Build history of the part. All positions in model axes, mm. A direction names the side the tool comes from. Round coordinates to 2 decimals unless told otherwise and drop trailing zeros. Loops run counter-clockwise (first coordinate to the right, second up) from the corner with the lowest first, then second, coordinate; pieces in that order, holes last. Notation, with made-up numbers: M -34,41 L -10,41 A24 ccw -10,67 Z; hole C 73,36 d11. An arc over 180 degrees is marked long. One line per item, written item: value.
```python
from build123d import *

# Parameters (mm, degrees)
SKETCH_2_W               = 50
SKETCH_2_H               = 4
EXTRUDE_2_DEPTH          = 22.5
SKETCH_15_R              = 1.4
EXTRUDE_8_DEPTH          = 5
SKETCH_3_W               = 30
SKETCH_3_H               = 20
EXTRUDE_4_DEPTH          = 20
EXTRUDE_9_DEPTH          = 17.5
EXTRUDE_10_DEPTH         = 15
CUT_EXTRUDE_1_REACH      = 58.089
SKETCH_19_R              = 2.1
SKETCH_20_R              = 2
CUT_EXTRUDE_2_DEPTH      = 10
CUT_EXTRUDE_3_DEPTH      = 70.524879929
CUT_EXTRUDE_3_DEPTH_BACK = 70.524879929


with BuildPart() as part:
    # 草圖2 → 填料-伸長2 (new, symmetric)
    with BuildSketch(Plane(origin=(0, 0, 0), x_dir=(0, 0, -1), z_dir=(1, 0, 0))):
        with Locations((25, 2)):
            Rectangle(SKETCH_2_W, SKETCH_2_H)
    extrude(amount=EXTRUDE_2_DEPTH, both=True)

    # 草圖15 → 填料-伸長8 (add)
    with BuildSketch(Plane(origin=(0, 4, 0), x_dir=(1, 0, 0), z_dir=(0, 1, 0))):
        with Locations(Location((17.5, 39.2, 0), (0, 0, 90))):
            Circle(SKETCH_15_R)
        with Locations(Location((17.5, 24.2, 0), (0, 0, 90))):
            Circle(SKETCH_15_R)
    extrude(amount=EXTRUDE_8_DEPTH)

    # 草圖3 → 填料-伸長4 (add)
    with BuildSketch(Plane(origin=(0, 4, 0), x_dir=(1, 0, 0), z_dir=(0, 1, 0))):
        with Locations((0, 10)):
            Rectangle(SKETCH_3_W, SKETCH_3_H)
    extrude(amount=EXTRUDE_4_DEPTH)

    # 草圖16 → 填料-伸長9 (add)
    with BuildSketch(Plane(origin=(0, 0, 0), x_dir=(-1, 0, 0), z_dir=(0, 0, -1))):
        with BuildLine():
            Line((-15, 24), (-15, 36.000002525))
            Line((-15, 36.000002525), (-6, 36.000002525))
            ThreePointArc((-6, 36.000002525), (-5.267141914, 33.146824473), (-3.25, 31.000002525))
            Line((-3.25, 31.000002525), (3.25, 31.000002525))
            ThreePointArc((3.25, 31.000002525), (5.267141914, 33.146824473), (6, 36.000002525))
            Line((6, 36.000002525), (15, 36.000002525))
            Line((15, 36.000002525), (15, 24))
            Line((15, 24), (-15, 24))
        make_face()
    extrude(amount=EXTRUDE_9_DEPTH)

    # 草圖18 → 填料-伸長10 (add, symmetric)
    with BuildSketch(Plane(origin=(0, 0, 0), x_dir=(0, 0, -1), z_dir=(1, 0, 0))):
        Polygon((17.5, 24), (28.5, 24), (28.5, 42.748788628), (27, 42.748788628), (27, 30.5), (17.5, 30.5), align=None)
    extrude(amount=EXTRUDE_10_DEPTH, both=True)

    # 草圖19 → 除料-伸長1 (cut, up to next)
    with BuildSketch(Plane(origin=(0, 0, -28.5), x_dir=(-1, 0, 0), z_dir=(0, 0, -1)), mode=Mode.PRIVATE) as cut_extrude_1_sk1:
        with Locations((0, 36.000002505)):
            Circle(SKETCH_19_R)
    cut_extrude_1_tool1 = extrude(cut_extrude_1_sk1.sketch, amount=-CUT_EXTRUDE_1_REACH, mode=Mode.PRIVATE) & part.part
    add(cut_extrude_1_tool1.solids().sort_by_distance((0, 36.000003, -28.5))[0], mode=Mode.SUBTRACT)

    # 草圖20 → 除料-伸長2 (cut)
    with BuildSketch(Plane(origin=(0, 36.000002525, 0), x_dir=(1, 0, 0), z_dir=(0, 1, 0))):
        with Locations(Location((-11.5, 8.75, 0), (0, 0, 180))):
            Circle(SKETCH_20_R)
        with Locations(Location((11.5, 8.75, 0), (0, 0, 180))):
            Circle(SKETCH_20_R)
    extrude(amount=-CUT_EXTRUDE_2_DEPTH, mode=Mode.SUBTRACT)

    # 草圖21 → 除料-伸長3 (cut, two sides: drawn at the far end of the back side and taken through both)
    with BuildSketch(Plane(origin=(0, 0, 0), x_dir=(0, 0, -1), z_dir=(1, 0, 0)).offset(-CUT_EXTRUDE_3_DEPTH_BACK)):
        Polygon((0, 0), (0, 27.945687573), (17.572849685, 27.945687573), (17.572849685, 46.39939524), (61.461395387, 46.39939524), (61.461395387, 0), align=None)
    extrude(amount=CUT_EXTRUDE_3_DEPTH + CUT_EXTRUDE_3_DEPTH_BACK, mode=Mode.SUBTRACT)


solid = part.part
```
Item 1: Slice it at B-B, the plane y = 34. Give the cut face in (x, z).
Check values:
outline: M -15,-17.5 L -5.65,-17.5 L -5.65,0 L -15,0 Z; M 5.65,-17.5 L 15,-17.5 L 15,0 L 5.65,0 Z; hole C -11.5,-8.75 d4; hole C 11.5,-8.75 d4
Item 2: Which spindle directions (+Z, -Z, +X, -X, +Y, -Y) get a long thin tool onto all of the face, cutting with end or side? Do faces 4 (the face through (15, 32, -9)), 5 (the face through (-0.2, 30.8, -17.5)), 6 (the face through (5.287, 33.183, -8.628)). Say none if no direction does.
Check values:
face 4: +Z, -Z, +X, +Y, -Y
face 5: -Z, +X, -X, +Y
face 6: +Z, -Z, +Y
Item 3: Slice it at A-A, the plane x = -11.5. Give the cut face in (y, z), and give its area (3 significant figures).
Check values:
outline: M 27.95,-17.57 L 30.5,-17.57 L 30.5,-17.5 L 36,-17.5 L 36,-10.75 L 27.95,-10.75 Z; M 27.95,-6.75 L 36,-6.75 L 36,0 L 27.95,0 Z
area: 109 mm2
Item 4: Drop flat-ended pins along their axis: P1, Ø2.5, axis at x = -11.5, z = -8.75, coming from the -Y side; P2, Ø1, axis at x = -4.5, z = -5.5, coming from the +Y side; P3, Ø1.7, axis at x = -4.5, y = 32.5, coming from the -Z side; P4, Ø7, axis at x = -1, z = -5.5, coming from the +Y side. Give the stop position or say it passes through.
Check values:
P1: passes through
P2: stops at y = 32.71
P3: stops at z = -17.5
P4: stops at y = 32.06
Item 5: Slice it at D-D, the plane y = 28.5. Give the cut face in (x, z), and give its area (3 significant figures).
Check values:
outline: M -15,-17.57 L 15,-17.57 L 15,0 L -15,0 Z; hole C -11.5,-8.75 d4; hole C 11.5,-8.75 d4
area: 502 mm2
Item 6: Pull direction Z, two halves, no side cores. Call faces 1 (the face through (-10.026, 32.029, -7.398)), 2 (the face through (0, 29, -17.573)), 3 (the face through (0, 31, -9)): pulls with the +Z half, pulls with the -Z half, needs draft (parallel to the pull), parting line crosses it, or undercut.
Check values:
face 1: undercut
face 2: pulls with the -Z half
face 3: needs draft
Item 7: Wall check: line 1 along Z through (x, y) = (11.5, 31.5); line 2 along X through (y, z) = (33.25, -9.5); line 3 along X through (y, z) = (31.75, -7.25). Give the ranges that are in metal, low to high.
Check values:
line 1: z = -17.5 to -10.75, -6.75 to 0
line 2: x = -15 to -13.35, -9.65 to -5.32, 5.32 to 9.65, 13.35 to 15
line 3: x = -15 to -12.82, -10.18 to -4.2, 4.2 to 10.18, 12.82 to 15
Item 8: Slice it at C-C, the plane z = -8.75. Give the cut face in (x, y).
Check values:
outline: M -15,27.95 L -13.5,27.95 L -13.5,36 L -15,36 Z; M -9.5,27.95 L 9.5,27.95 L 9.5,36 L 6,36 A5.92 cw 3.25,31 L -3.25,31 A5.92 cw -6,36 L -9.5,36 Z; M 13.5,27.95 L 15,27.95 L 15,36 L 13.5,36 Z
